Build history of the part. All positions in model axes, mm. Face numbers are marked on the shaded views. A direction names the side the tool comes from. Give positions to 0.01 mm unless a question says otherwise; leave off trailing zeros. Order: outer loops, then holes, each group sorted by start corner. A loop starts at its lowest first (then second) coordinate and runs counter-clockwise, first axis right, second up. Notation, with made-up numbers: (85.25, -10) -> (115.25, -10) arc R21 cw to (115.25, 5) -> close; hole circle Ø4 at (-35.75, 3). An arc over 180 degrees is marked (long way). Use a Markdown table: item, result. Add a question column.
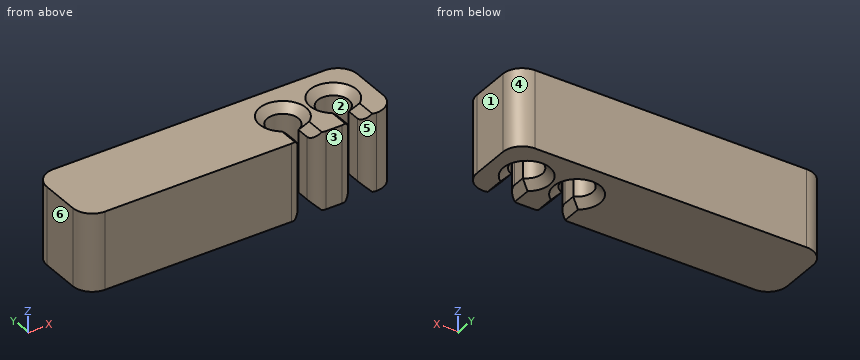
```python
from build123d import *

# Parameters (mm, degrees)
F0_W     = 80
F0_H     = 20
F1_DEPTH = 20
F3_DEPTH = 20.001
F4_R     = 4
F5_DEPTH = 20.001
F6_SIZE  = 2
F7_R     = 3
F8_R     = 4.99999


# Not quite as in the source:
# - a fillet or chamfer is up to 0.001 mm smaller than in the source, because OpenCascade refuses the exact size


with BuildPart() as f1:
    # F0 (on Top) → F1 (new body)
    with BuildSketch(Plane.XY):
        Rectangle(F0_W, F0_H)
    extrude(amount=F1_DEPTH)

    # F2 (on face) → F3 (cut, through all)
    with BuildSketch(Plane.XY.offset(20)):
        with BuildLine():
            Line((29, -10), (32, -10))
            Line((32, -10), (32, 0))
            ThreePointArc((32, 0), (30.5, 1.5), (29, 0))
            Line((29, 0), (29, -10))
        make_face()
        with BuildLine():
            Line((16, -10), (19, -10))
            Line((19, -10), (19, 0))
            ThreePointArc((19, 0), (17.5, 1.5), (16, 0))
            Line((16, 0), (16, -10))
        make_face()
    extrude(amount=-F3_DEPTH, mode=Mode.SUBTRACT)

    # F4 (on face) → F5 (cut, through all)
    with BuildSketch(Plane.XY.offset(20)):
        with Locations((17.5, 0)):
            Circle(F4_R)
        with Locations((30.5, 0)):
            Circle(F4_R)
    extrude(amount=-F5_DEPTH, mode=Mode.SUBTRACT)

    # F6
    f6_edges = [f1.edges().sort_by_distance(p)[0] for p in [
        (17.5, 4, 20),
        (30.5, 4, 20),
        (17.5, 4, 0),
        (30.5, 4, 0),
        (16, -6.85405, 20),
        (19, -6.85405, 20),
        (29, -6.85405, 20),
        (32, -6.85405, 20),
        (16, -6.85405, 0),
        (19, -6.85405, 0),
        (29, -6.85405, 0),
        (32, -6.85405, 0),
    ]]
    chamfer(f6_edges, length=F6_SIZE)

    # F7
    f7_edges = [f1.edges().sort_by_distance(p)[0] for p in [
        (19, -10, 10),
        (29, -10, 10),
        (32, -10, 10),
        (16, -10, 10),
    ]]
    fillet(f7_edges, radius=F7_R)

    # F8 (radius 5 in the source; OpenCascade refuses exactly that, so slightly less here)
    f8_edges = [f1.edges().sort_by_distance(p)[0] for p in [
        (40, -10, 10),
        (40, 10, 10),
        (-40, 10, 10),
        (-40, -10, 10),
    ]]
    fillet(f8_edges, radius=F8_R)


solid = f1.part
```
(1) Band-saw the part on C-C on x = 30.5. Give the cut face in (y, z), plus the area to 3 significant figures.
(2) Mould opens along Y. For the marked faces 1, 2, 3 and 4 say: released by +Y, released by -Y, zero draft, split by the parting line, or undercut.
(3) Band-saw the part on B-B on y = 0. Give the cut face in (x, z), plus the area to 3 significant figures.
(4) Tool access for the marked faces 5 and 6: list every direction of +Z, -Z, +X, -X, +Y, -Y with a clear straight run to the whole face (end or side of a thin tool).
(5) Band-saw the part on D-D on y = 8.25. Give the cut face in (x, z), plus the area to 3 significant figures.
(6) Wall check: probe 1 along X at (y, z) = (0, 14.25); probe 2 along X at (y, z) = (-2.5, 4); probe 3 along Y at (x, z) = (30.5, 5.5). Give the ranges that are in metal, low to high.
(7) Pin check, flat tip, straight feed: pin 1 Ø6.5 at (x, y) = (30.5, 0) entering from -Z. Stop position of the tip, or through.
Response:
| question | item | result |
|---|---|---|
| 1 | outline | (4, 2) -> (6, 0) -> (10, 0) -> (10, 20) -> (6, 20) -> (4, 18) -> close |
| 1 | area | 116 mm² |
| 2 | face 1 | zero draft |
| 2 | face 2 | undercut |
| 2 | face 3 | released by -Y |
| 2 | face 4 | released by +Y |
| 3 | outline | (-40, 0) -> (11.5, 0) -> (13.5, 2) -> (13.5, 18) -> (11.5, 20) -> (-40, 20) -> close; (21.5, 2) -> (23.5, 0) -> (24.5, 0) -> (26.5, 2) -> (26.5, 18) -> (24.5, 20) -> (23.5, 20) -> (21.5, 18) -> close; (34.5, 2) -> (36.5, 0) -> (40, 0) -> (40, 20) -> (36.5, 20) -> (34.5, 18) -> close |
| 3 | area | 1,260 mm² |
| 4 | face 5 | +Z, -Z, -Y |
| 4 | face 6 | +Z, -Z, -X, +Y, -Y |
| 5 | outline | (-38.8, 0) -> (38.8, 0) -> (38.8, 20) -> (-38.8, 20) -> close |
| 5 | area | 1,550 mm² |
| 6 | probe 1 | x = -40 to 13.5, 21.5 to 26.5, 34.5 to 40 |
| 6 | probe 2 | x = -40 to 14.38, 20.62 to 27.38, 33.62 to 40 |
| 6 | probe 3 | y = 4 to 10 |
| 7 | pin 1 | passes through |
